Verification items for the finished model (mm, model axes). Face numbers are marked on the shaded views. A direction names the side the tool comes from. Round coordinates to 2 decimals unless told otherwise and drop trailing zeros. Loops run counter-clockwise (first coordinate to the right, second up) from the corner with the lowest first, then second, coordinate; pieces in that order, holes last. Notation, with made-up numbers: (-6.5, -33.5) -> (10.5, -33.5) arc R11 ccw to (10.5, -19.5) -> close; hole circle Ø10 at (3, -17.75). An arc over 180 degrees is marked (long way). Write item = value, one per line. Start each with the question number.
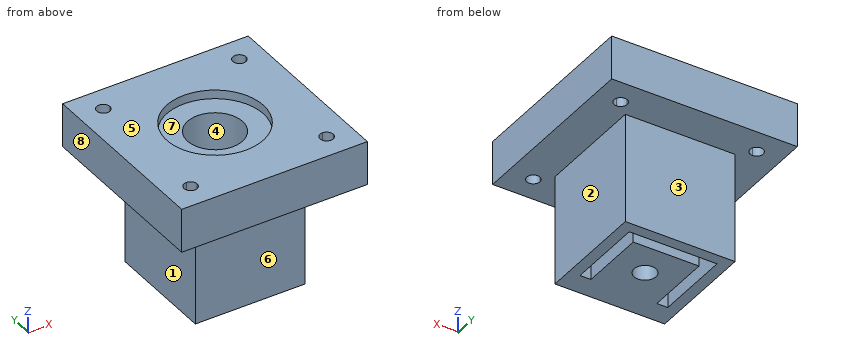
```python
from build123d import *

# Parameters (mm, degrees)
F0_W     = 42.3
F0_H     = 42.3
F0_R     = 7.5
F0_R_2   = 2.5
F1_DEPTH = 10
F2_R     = 11
F3_DEPTH = 2
F4_W     = 25
F4_H     = 25
F4_W_2   = 15
F4_H_2   = 15
F4_R     = 2.5
F5_DEPTH = 25
F6_R     = 6.25
F7_DEPTH = 10


with BuildPart() as f1:
    # F0 (on Top) → F1 (new body)
    with BuildSketch(Plane.XY):
        Rectangle(F0_W, F0_H)
        with BuildLine():
            Line((14, -15.5), (-14, -15.5))
            ThreePointArc((-14, -15.5), (-16.5606601718, -16.5606601718), (-15.5, -14))
            Line((-15.5, -14), (-15.5, 14))
            ThreePointArc((-15.5, 14), (-16.5606601718, 16.5606601718), (-14, 15.5))
            Line((-14, 15.5), (14, 15.5))
            ThreePointArc((14, 15.5), (15.5, 17), (17, 15.5))
            ThreePointArc((17, 15.5), (16.5606601718, 14.4393398282), (15.5, 14))
            Line((15.5, 14), (15.5, -14))
            ThreePointArc((15.5, -14), (16.5606601718, -14.4393398282), (17, -15.5))
            ThreePointArc((17, -15.5), (15.5, -17), (14, -15.5))
        make_face(mode=Mode.SUBTRACT)
        with BuildLine():
            ThreePointArc((-15.5, -14), (-14.4393398282, -14.4393398282), (-14, -15.5))
            Line((-14, -15.5), (14, -15.5))
            ThreePointArc((14, -15.5), (14.4393398282, -14.4393398282), (15.5, -14))
            Line((15.5, -14), (15.5, 14))
            ThreePointArc((15.5, 14), (14.4393398282, 14.4393398282), (14, 15.5))
            Line((14, 15.5), (-14, 15.5))
            ThreePointArc((-14, 15.5), (-14.4393398282, 14.4393398282), (-15.5, 14))
            Line((-15.5, 14), (-15.5, -14))
        make_face()
        Circle(F0_R, mode=Mode.SUBTRACT)
        Circle(F0_R)
        Circle(F0_R_2, mode=Mode.SUBTRACT)
    extrude(amount=F1_DEPTH)

    # F2 (on face) → F3 (cut)
    with BuildSketch(Plane.XY.offset(10)):
        Circle(F2_R)
    extrude(amount=-F3_DEPTH, mode=Mode.SUBTRACT)

    # F4 (on face) → F5 (join)
    with BuildSketch(Plane(origin=(0, 0, 0), x_dir=(1, 0, 0), z_dir=(0, 0, -1))):
        Rectangle(F4_W, F4_H)
        Polygon((-10, 7.5), (-10, 10), (10, 10), (10, 7.5), (10, -10), (-10, -10), align=None, mode=Mode.SUBTRACT)
        Rectangle(F4_W_2, F4_H_2)
        Circle(F4_R, mode=Mode.SUBTRACT)
        Polygon((10, 10), (-10, 10), (-10, 7.5), (-7.5, 7.5), (7.5, 7.5), (10, 7.5), align=None)
    extrude(amount=F5_DEPTH)

    # F6 (on face) → F7 (cut)
    with BuildSketch(Plane.XY.offset(8)):
        Circle(F6_R)
    extrude(amount=-F7_DEPTH, mode=Mode.SUBTRACT)


solid = f1.part
```
(1) Scan lines: line 1 (X direction, y = 15.5, z = 7); line 2 (X direction, y = 0, z = -12.25). Record each from-to range of solid material in increasing order. Write a range as [from, to].
(2) Section check D-D on y = -3.5. Enter the section's corners in (x, z).
(3) Access from +Z, -Z, +X, -X, +Y, -Y to the whole of each face (thin tool, end or side, straight path). Record for the marked faces 1, 2, 3, 4 and 5.
(4) Depth check by flat-ended pin: pin 1 Ø6.5 at (x, y) = (1.5, 4) entering from +Z; pin 2 Ø0.8 at (x, z) = (-9, -8.5) entering from +Y; pin 3 Ø5 at (y, z) = (4, -12) entering from -X. Enter the tip coordinate at first touch or a pass-through.
(5) Draft check along X on the marked faces 6, 7 and 8. Enter one of: +X half, -X half, draft (parallel to the pull), parting line (faces both ways), or undercut.
(6) Section check B-B on z = -13. Enter the section's corners in (x, y), then the cut area to 3 significant figures.
(7) Section check C-C on z = 7. Enter the section's corners in (x, y).
(8) Section check A-A on x = 0. Enter the section's corners in (y, z), then the cut area to 4 significant figures.
Computed values:
q1.line_1 = [-21.15, -17], [-14, 14], [17, 21.15]
q1.line_2 = [-12.5, -10], [-7.5, -2.5], [2.5, 7.5], [10, 12.5]
q2.outline = (-21.15, 0) -> (-12.5, 0) -> (-12.5, -25) -> (-10, -25) -> (-10, 0) -> (-7.5, 0) -> (-7.5, -25) -> (7.5, -25) -> (7.5, 0) -> (10, 0) -> (10, -25) -> (12.5, -25) -> (12.5, 0) -> (21.15, 0) -> (21.15, 10) -> (10.43, 10) -> (10.43, 8) -> (5.18, 8) -> (5.18, -2) -> (-5.18, -2) -> (-5.18, 8) -> (-10.43, 8) -> (-10.43, 10) -> (-21.15, 10) -> close
q3.face_1 = -Z, -X, +Y, -Y
q3.face_2 = -Z, +X, +Y, -Y
q3.face_3 = -Z, +X, -X, +Y
q3.face_4 = +Z
q3.face_5 = +Z, +X, -X, +Y, -Y
q4.pin_1 = 8
q4.pin_2 = 12.5
q4.pin_3 = -12.5
q5.face_6 = draft
q5.face_7 = undercut
q5.face_8 = -X half
q6.outline = (-12.5, -12.5) -> (12.5, -12.5) -> (12.5, 12.5) -> (-12.5, 12.5) -> close; hole (-10, -7.5) -> (-7.5, -7.5) -> (-7.5, 7.5) -> (7.5, 7.5) -> (7.5, -7.5) -> (10, -7.5) -> (10, 10) -> (-10, 10) -> close; hole circle Ø5 at (0, 0)
q6.area = 480 mm²
q7.outline = (-21.15, -21.15) -> (21.15, -21.15) -> (21.15, 21.15) -> (-21.15, 21.15) -> close; hole circle Ø3 at (-15.5, -15.5); hole circle Ø3 at (-15.5, 15.5); hole circle Ø12.5 at (0, 0); hole circle Ø3 at (15.5, -15.5); hole circle Ø3 at (15.5, 15.5)
q8.outline = (-21.15, 0) -> (-12.5, 0) -> (-12.5, -25) -> (-2.5, -25) -> (-2.5, -2) -> (-6.25, -2) -> (-6.25, 8) -> (-11, 8) -> (-11, 10) -> (-21.15, 10) -> close; (2.5, -25) -> (7.5, -25) -> (7.5, 0) -> (10, 0) -> (10, -25) -> (12.5, -25) -> (12.5, 0) -> (21.15, 0) -> (21.15, 10) -> (11, 10) -> (11, 8) -> (6.25, 8) -> (6.25, -2) -> (2.5, -2) -> close
q8.area = 701.5 mm²
